The model under review builds one solid part; all positions refer to its coordinate system, in mm. Face numbers are marked on the shaded views. A direction names the side the tool comes from. Coordinates: 2 decimals unless noted, no trailing zeros. Order: outer loops, then holes, each group sorted by start corner. A loop starts at its lowest first (then second) coordinate and runs counter-clockwise, first axis right, second up. Notation, with made-up numbers: M -12,-23.5 L 9,-23.5 A14 cw 9,2.5 Z; hole C 46.5,45 d6. An arc over 180 degrees is marked long. Answer in a Markdown table with one row per item.
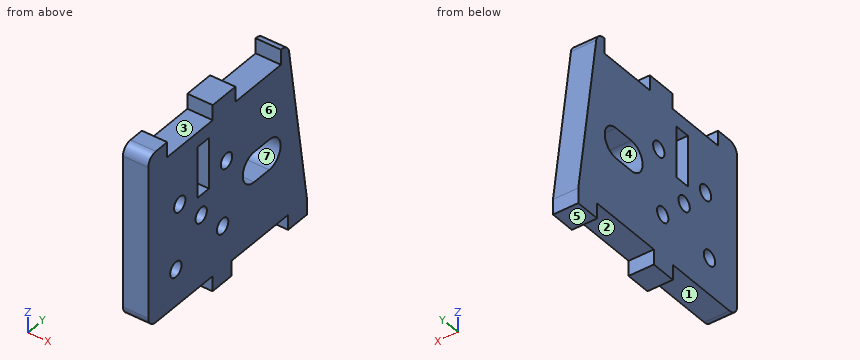
from build123d import *

# Parameters (mm, degrees)
SKETCH1_R           = 1.5
BOSS_EXTRUDE1_DEPTH = 5
SKETCH2_W           = 3
SKETCH2_H           = 12.05
SKETCH2_W_2         = 10.1
SKETCH2_H_2         = 3.05
CUT_EXTRUDE1_DEPTH  = 35.770677301
CUT_EXTRUDE3_DEPTH  = 10
FILLET1_R           = 2


with BuildPart() as part:
    # Sketch1 → Boss-Extrude1 (new body)
    with BuildSketch(Plane(origin=(0, 0, 0), x_dir=(0, 0, -1), z_dir=(1, 0, 0))):
        Polygon((17, 28), (17, 23), (14, 23), (14, 8), (17, 8), (17, 3), (14, 3), (14, -14), (-20, -14), (-20, 23), (14, 28), align=None)
        with Locations((-6.733876165, 6.701112728)):
            Circle(SKETCH1_R, mode=Mode.SUBTRACT)
        with Locations((-5.643042298, -5.67063256)):
            Circle(SKETCH1_R, mode=Mode.SUBTRACT)
        with Locations((6.733876165, -6.701112728)):
            Circle(SKETCH1_R, mode=Mode.SUBTRACT)
        with Locations((5.643042298, 5.67063256)):
            Circle(SKETCH1_R, mode=Mode.SUBTRACT)
        Circle(SKETCH1_R, mode=Mode.SUBTRACT)
    extrude(amount=BOSS_EXTRUDE1_DEPTH)

    # Sketch2 → Cut-Extrude1 (cut, through all)
    with BuildSketch(Plane(origin=(5, 0, 0), x_dir=(0, 0, -1), z_dir=(1, 0, 0))):
        with Locations((-18.5, 15.075)):
            Rectangle(SKETCH2_W, SKETCH2_H)
        with Locations((-9.05, 0.525)):
            Rectangle(SKETCH2_W_2, SKETCH2_H_2)
        with Locations((-18.5, -2.975)):
            Rectangle(SKETCH2_W, SKETCH2_H)
    extrude(amount=-CUT_EXTRUDE1_DEPTH, mode=Mode.SUBTRACT)

    # Sketch4 → Cut-Extrude3 (cut)
    with BuildSketch(Plane(origin=(5, 0, 0), x_dir=(0, 0, -1), z_dir=(1, 0, 0))):
        with BuildLine():
            Line((-4, 18), (-4, 14))
            ThreePointArc((-4, 14), (-1, 11), (2, 14))
            Line((2, 14), (2, 18))
            ThreePointArc((2, 18), (-1, 21), (-4, 18))
        make_face()
    extrude(amount=-CUT_EXTRUDE3_DEPTH, mode=Mode.SUBTRACT)

    # Fillet1
    fillet1_edges = [part.edges().sort_by_distance(p)[0] for p in [
        (2.5, -14, -14),
        (2.5, -14, 20),
        (2.5, 23, 20),
    ]]
    fillet(fillet1_edges, radius=FILLET1_R)


solid = part.part
(1) To check wall thickness, follow line 1 (Y direction, x = 1.2, z = 1); line 2 (Z direction, x = 0.7, y = 16.5); line 3 (Z direction, x = 2.5, y = 6.5). State the ranges of each line that lie inside material, in increasing order. Write a range as [from, to].
Report:
| item | result |
|---|---|
| line 1 | [-14, -1.12], [1.12, 11], [21, 25.79] |
| line 2 | [-14, -2], [4, 17] |
| line 3 | [-17, -6.89], [-4.39, 5.25], [8.22, 20] |
(2) Take a section at D-D (z = 6). Write out the cut boundary in (x, y).
Report:
| item | result |
|---|---|
| outline | M 0,-14 L 5,-14 L 5,-7.13 L 0,-7.13 Z; M 0,-4.21 L 5,-4.21 L 5,-1 L 0,-1 Z; M 0,2.05 L 5,2.05 L 5,5.39 L 0,5.39 Z; M 0,8.01 L 5,8.01 L 5,25.06 L 0,25.06 Z |
(3) Take a section at A-A (y = 15.5). Write out the cut boundary in (x, z).
Report:
| item | result |
|---|---|
| outline | M 0,-14 L 5,-14 L 5,-2 L 0,-2 Z; M 0,4 L 5,4 L 5,17 L 0,17 Z |
(4) Take a section at C-C (z = -0.5). Write out the cut boundary in (x, y), then the cut area to 3 significant figures.
Report:
| item | result |
|---|---|
| outline | M 0,-14 L 5,-14 L 5,-1.41 L 0,-1.41 Z; M 0,1.41 L 5,1.41 L 5,11.4 L 0,11.4 Z; M 0,20.6 L 5,20.6 L 5,26.01 L 0,26.01 Z |
| area | 140 mm^2 |
(5) Machinability: for the marked faces 1, 2, 3 and 4, which of the approach directions +Z, -Z, +X, -X, +Y, -Y give a long, thin tool a straight path to every point of the face, cutting with its end or side? Answer none if there is none.
Report:
| item | result |
|---|---|
| face 1 | -Z, +X, -X, -Y |
| face 2 | -Z, +X, -X |
| face 3 | +Z, +X, -X |
| face 4 | +X, -X |
(6) Insertion check: P1, Ø0.9, axis at x = 2, z = 19, coming from the -Y side; P2, Ø2.5, axis at x = 2, z = 19, coming from the +Y side; P3, Ø0.9, axis at x = 2, z = -15, coming from the -Y side; P4, Ø2.5, axis at y = 6.7, z = 6.73, coming from the -X side. Each pin has a flat end and moves straight along its axis. Give the tip position at first contact, or say it passes through.
Report:
| item | result |
|---|---|
| P1 | y = -13.92 |
| P2 | y = 23.33 |
| P3 | y = 3 |
| P4 | through |
(7) The part is to be moulded in two halves that separate along Z. For the marked faces 5, 6 and 7, say which applies: +Z half, -Z half, draft (parallel to the pull), parting line (faces both ways), or undercut.
Report:
| item | result |
|---|---|
| face 5 | -Z half |
| face 6 | draft |
| face 7 | undercut |
(8) Take a section at B-B (y = 0). Write out the cut boundary in (x, z).
Report:
| item | result |
|---|---|
| outline | M 0,-14 L 5,-14 L 5,-1.5 L 0,-1.5 Z; M 0,1.5 L 5,1.5 L 5,4 L 0,4 Z; M 0,14.1 L 5,14.1 L 5,17 L 0,17 Z |
